```python
from build123d import *

# Parameters (mm, degrees)
F0_R     = 8.5
F1_DEPTH = 4
F2_R     = 5
F3_DEPTH = 100


with BuildPart() as f1:
    # F0 (on Top) → F1 (new body)
    with BuildSketch(Plane.XY):
        Circle(F0_R)
    extrude(amount=F1_DEPTH)

    # F2 (on Top) → F3 (join)
    with BuildSketch(Plane.XY):
        Circle(F2_R)
    extrude(amount=F3_DEPTH)

    # F4 (on Right) → F5 (revolve)
    with BuildSketch(Plane.YZ):
        with BuildLine():
            Line((0, 104.582576), (0, 100))
            Line((0, 100), (5, 100))
            ThreePointArc((5, 100), (4.1833, 102.738613), (2, 104.582576))
            Line((2, 104.582576), (0, 104.582576))
        make_face()
        with BuildLine():
            ThreePointArc((0, 105), (1.021548, 104.894532), (2, 104.582576))
            Line((2, 104.582576), (2, 109.582576))
            Line((2, 109.582576), (0, 109.582576))
            Line((0, 109.582576), (0, 105))
        make_face()
        with BuildLine():
            Line((0, 105), (0, 104.582576))
            Line((0, 104.582576), (2, 104.582576))
            ThreePointArc((2, 104.582576), (1.021548, 104.894532), (0, 105))
        make_face()
    revolve(axis=Axis((0, 0, 104.791288), (0, 0, -1)))


solid = f1.part
```
Source: CAD feature listing. Evaluate the final solid. Frame: model axes, mm. A direction names the side the tool comes from. Round coordinates to 2 decimals unless told otherwise and drop trailing zeros. Loops run counter-clockwise (first coordinate to the right, second up) from the corner with the lowest first, then second, coordinate; pieces in that order, holes last. Notation, with made-up numbers: M 62.5,42 L 117.5,42 A4 ccw 117.5,47 Z; hole C 0.5,62 d10. An arc over 180 degrees is marked long. Use a Markdown table: item, result. Add a question column.
1. Contact query for flat-ended pins moving along their axis: P1, Ø4, axis at x = -5.5, y = -6, coming from the -Z side; P2, Ø3, axis at x = 1.5, z = 38.5, coming from the +Y side; P3, Ø6, axis at y = 5, z = 80.5, coming from the +X side; P4, Ø8, axis at x = 6.5, z = 61, coming from the +Y side. Output: stop coordinate, or through.
2. Line query: line 1 (Z direction, x = 6.5, y = -2.75); line 2 (X direction, y = 0.75, z = 52.5); line 3 (Y direction, x = 3.25, z = 91). Output: solid intervals per line, ascending.
3. Section query A-A on z = 92. Return the cut outline in (x, y).
4. Reachability of faces 1 (the flat face through (0, 0, 109.583)), 2 (the flat face through (4, -4, 4)) from +Z, -Z, +X, -X, +Y, -Y: full face, straight path, thin tool, end or side. Return the list, or none.
5. Section query B-B on y = 6.25. Return the cut outline in (x, z).
Reported:
| question | item | result |
|---|---|---|
| 1 | P1 | stops at z = 0 |
| 1 | P2 | stops at y = 5 |
| 1 | P3 | stops at x = 4.58 |
| 1 | P4 | stops at y = 4.33 |
| 2 | line 1 | z = 0 to 4 |
| 2 | line 2 | x = -4.94 to 4.94 |
| 2 | line 3 | y = -3.8 to 3.8 |
| 3 | outline | C 0,0 d10 |
| 4 | face 1 | +Z, +X, -X, +Y, -Y |
| 4 | face 2 | +Z |
| 5 | outline | M -5.76,0 L 5.76,0 L 5.76,4 L -5.76,4 Z |
